```python
from build123d import *

# Parameters (mm, degrees)
F0_W     = 72
F0_H     = 72
F1_DEPTH = 3
F2_W     = 52
F2_H     = 72
F3_DEPTH = 20
F5_D     = 4.5
F7_D     = 4.5
F8_R     = 5
F9_R     = 3


with BuildPart() as f1:
    # F0 (on Top) → F1 (new body)
    with BuildSketch(Plane.XY):
        Rectangle(F0_W, F0_H)
    extrude(amount=F1_DEPTH)

    # F2 (on face) → F3 (join)
    with BuildSketch(Plane.XY.offset(3)):
        Rectangle(F2_W, F2_H)
    extrude(amount=F3_DEPTH)

    # F5 (through all)
    with Locations(Plane.XY.offset(3)):
        with Locations((32, 32), (32, 16), (32, 0), (32, -16), (32, -32)):
            Hole(F5_D / 2)

    # F7 (through all)
    with Locations(Plane.XY.offset(3)):
        with Locations((-32, 32), (-32, 16), (-32, 0), (-32, -16), (-32, -32)):
            Hole(F7_D / 2)

    # F8
    f8_edges = [f1.edges().sort_by_distance(p)[0] for p in [
        (-36, 36, 1.5),
        (-36, -36, 1.5),
        (36, -36, 1.5),
        (36, 36, 1.5),
    ]]
    fillet(f8_edges, radius=F8_R)

    # F9
    f9_edges = [f1.edges().sort_by_distance(p)[0] for p in [
        (-26, -36, 13),
        (26, -36, 13),
        (0, -36, 23),
        (-26, 0, 23),
        (0, 36, 23),
        (26, 0, 23),
        (26, 36, 13),
        (-26, 36, 13),
    ]]
    fillet(f9_edges, radius=F9_R)


solid = f1.part
```
Source: CAD feature listing. Evaluate the final solid. Frame: model axes, mm. A direction names the side the tool comes from. Give positions to 0.01 mm unless a question says otherwise; leave off trailing zeros. Write each loop counter-clockwise with the first axis right and the second up, starting at its lowest first coordinate (ties: lowest second). Pieces come first, ordered by that corner, then holes. Notation, with made-up numbers: (34, 49) - (64, 49) arc R9 cw to (64, 57) - close; hole circle Ø3 at (70.5, 63). An arc over 180 degrees is marked (long way). One line per item, written item: value. Start each with the question number.
Q1. Set-up query: faces 1 (the face through (25.1, 35.14, 11.62)), 2 (the face through (-25.1, -35.14, 11.62)), 3 (the face through (-25.1, 35.14, 11.62)). Return all of +Z, -Z, +X, -X, +Y, -Y with unobstructed straight access to the full face (end or side cutting, diameter ignored); none if empty.
Q2. Material intervals for probe 1 along Y at (x, z) = (32, 1.55); probe 2 along X at (y, z) = (14, 12); probe 3 along Z at (x, y) = (-30, 14), sorted ascending. Write a range as from..to.
Q3. First-contact query: pin 1 Ø7 at (x, y) = (-32, -16) entering from +Z; pin 2 Ø14.5 at (x, y) = (32.5, 15) entering from +Z; pin 3 Ø4 at (y, z) = (-27, 16) entering from -X. Flat tips, straight axial feed; report the tip coordinate or a pass-through.
Q4. Draft query along Y for faces 4 (the face through (-35, -34, 2)), 5 (the face through (-34.08, -16.86, 1.48)), 6 (the face through (25.1, 0.46, 22.14)), 7 (the face through (0.32, 35.14, 22.1)). Return one class per face: +Y half, -Y half, draft (parallel to the pull), parting line (faces both ways), or undercut.
Q5. Section query D-D, the plane y = 26. Return the cut outline in (x, z), then the cut area to 3 significant figures.
Q6. Section query A-A, the plane y = 0. Return the cut outline in (x, z), then the cut area to 3 significant figures.
Q7. Section query B-B, the plane z = 1.5. Count the separate pieces of the cut face and the enclosed holes in it, then the cut area to 3 significant figures.
Q8. Section query C-C, the plane x = -32. Return the cut outline in (y, z), then the cut area to 3 significant figures.
Answer:
1. face 1: +Z, +X, +Y
1. face 2: +Z, -X, -Y
1. face 3: +Z, -X, +Y
2. probe 1: y = -35.9..-34.25, -29.75..-18.25, -13.75..-2.25, 2.25..13.75, 18.25..29.75, 34.25..35.9
2. probe 2: x = -26..26
2. probe 3: z = 0..3
3. pin 1: stops at z = 3
3. pin 2: stops at z = 21.98
3. pin 3: stops at x = -26
4. face 4: -Y half
4. face 5: undercut
4. face 6: draft
4. face 7: +Y half
5. outline: (-36, 0) - (36, 0) - (36, 3) - (26, 3) - (26, 20) arc R3 ccw to (23, 23) - (-23, 23) arc R3 ccw to (-26, 20) - (-26, 3) - (-36, 3) - close
5. area: 1,250 mm2
6. outline: (-36, 0) - (-34.25, 0) - (-34.25, 3) - (-36, 3) - close; (-29.75, 0) - (29.75, 0) - (29.75, 3) - (26, 3) - (26, 20) arc R3 ccw to (23, 23) - (-23, 23) arc R3 ccw to (-26, 20) - (-26, 3) - (-29.75, 3) - close; (34.25, 0) - (36, 0) - (36, 3) - (34.25, 3) - close
6. area: 1,230 mm2
7. separate pieces: 1
7. enclosed holes: 10
7. area: 5,000 mm2
8. outline: (-35.9, 0) - (-34.25, 0) - (-34.25, 3) - (-35.9, 3) - close; (-29.75, 0) - (-18.25, 0) - (-18.25, 3) - (-29.75, 3) - close; (-13.75, 0) - (-2.25, 0) - (-2.25, 3) - (-13.75, 3) - close; (2.25, 0) - (13.75, 0) - (13.75, 3) - (2.25, 3) - close; (18.25, 0) - (29.75, 0) - (29.75, 3) - (18.25, 3) - close; (34.25, 0) - (35.9, 0) - (35.9, 3) - (34.25, 3) - close
8. area: 148 mm2
